Read the model definition and answer for the solid it produces. Units are mm, in the model's axes. A direction names the side the tool comes from. Coordinates: 2 decimals unless noted, no trailing zeros. Loops run counter-clockwise (first coordinate to the right, second up) from the corner with the lowest first, then second, coordinate; pieces in that order, holes last.
from build123d import *

# Parameters (mm, degrees)
F0_W     = 35.56
F0_H     = 35.56
F0_R     = 1.016
F0_W_2   = 24.13
F0_H_2   = 24.13
F1_DEPTH = 3.175


with BuildPart() as f1:
    # F0 (on Top) → F1 (new body)
    with BuildSketch(Plane.XY):
        Rectangle(F0_W, F0_H)
        with Locations((-14.986, 0)):
            Circle(F0_R, mode=Mode.SUBTRACT)
        Rectangle(F0_W_2, F0_H_2, mode=Mode.SUBTRACT)
        with Locations((14.986, 0)):
            Circle(F0_R, mode=Mode.SUBTRACT)
    extrude(amount=F1_DEPTH)


solid = f1.part
Item 1: A cutting plane is placed at A-A on y = 0. Determine the outline of the cut face in (x, z) (3 decimals).
Numbers:
outline: (-17.78, 0) - (-16.002, 0) - (-16.002, 3.175) - (-17.78, 3.175) - close; (-13.97, 0) - (-12.065, 0) - (-12.065, 3.175) - (-13.97, 3.175) - close; (12.065, 0) - (13.97, 0) - (13.97, 3.175) - (12.065, 3.175) - close; (16.002, 0) - (17.78, 0) - (17.78, 3.175) - (16.002, 3.175) - close
Item 2: Find the intervals of material crossed by line 1 along Y through (x, z) = (-5, 1.1) (3 decimals); line 2 along Y through (x, z) = (15, 2.3), in increasing order.
Numbers:
line 1: y = -17.78 to -12.065, 12.065 to 17.78
line 2: y = -17.78 to -1.02, 1.02 to 17.78
Item 3: Given pin 1 (6 mm diameter, centred on x = 13, y = -2.5, fed in from -Z), flat-ended and moving along its own axis, determine where the tip first touches the part or whether it passes through.
Numbers:
pin 1: stops at z = 0
Item 4: A cutting plane is placed at B-B on x = -1.5. Determine the outline of the cut face in (y, z) (3 decimals), then the cut area to 3 significant figures.
Numbers:
outline: (-17.78, 0) - (-12.065, 0) - (-12.065, 3.175) - (-17.78, 3.175) - close; (12.065, 0) - (17.78, 0) - (17.78, 3.175) - (12.065, 3.175) - close
area: 36.3 mm2
Item 5: A cutting plane is placed at D-D on z = 0.95. Determine the outline of the cut face in (x, y) (3 decimals).
Numbers:
outline: (-17.78, -17.78) - (17.78, -17.78) - (17.78, 17.78) - (-17.78, 17.78) - close; hole circle Ø2.032 at (-14.986, 0); hole (-12.065, -12.065) - (12.065, -12.065) - (12.065, 12.065) - (-12.065, 12.065) - close; hole circle Ø2.032 at (14.986, 0)
Item 6: Which of the six approach directions +Z, -Z, +X, -X, +Y, -Y give full straight-line access (tool end or side, diameter ignored) to faces 5 (the face through (0, 17.78, 2)), 6 (the face through (0, -12.065, 2))?
Numbers:
face 5: +Z, -Z, +X, -X, +Y
face 6: +Z, -Z
Item 7: Determine the mould class of faces 1 (the face through (-17.78, 0, 2)), 2 (the face through (12.065, 0, 2)), 3 (the face through (17.78, 0, 2)), 4 (the face through (0, -17.78, 2)) for opening direction X: released by +X, released by -X, zero draft, split by the parting line, or undercut.
Numbers:
face 1: released by -X
face 2: undercut
face 3: released by +X
face 4: zero draft
